Here's the drawing with two shaded views (mm, measured from the low corner). I have some questions. Coordinates: 2 decimals unless noted, no trailing zeros. Order: outer loops, then holes, each group sorted by start corner. A loop starts at its lowest first (then second) coordinate and runs counter-clockwise, first axis right, second up. Notation, with made-up numbers: (12, 28.5) - (56, 28.5) arc R5 cw to (56, 37.5) - close; hole circle Ø3 at (-33.5, 2). An arc over 180 degrees is marked (long way). Answer as a JSON object with one key per item and string values. Group by question number.
(1) Imagine slicing it at A-A, the plane x = 33.5. Write out the boundary of the cut face in (y, z).
(2) Will these pins go through, and if not, where does the flat tip stop? P1, Ø0.7, axis at x = 33.5, z = 7.6, coming from the -Y side; P2, Ø0.6, axis at x = 33.5, z = 30, coming from the -Y side.
(3) Imagine slicing it at B-B, the plane z = 30.4. Write out the boundary of the cut face in (x, y).
(4) Please list where these lines run through material, in increasing order: probe 1 along X at (y, z) = (0.65, 30.4); probe 2 along X at (y, z) = (1.8, 7.6); probe 3 along Z at (x, y) = (33.5, 1).
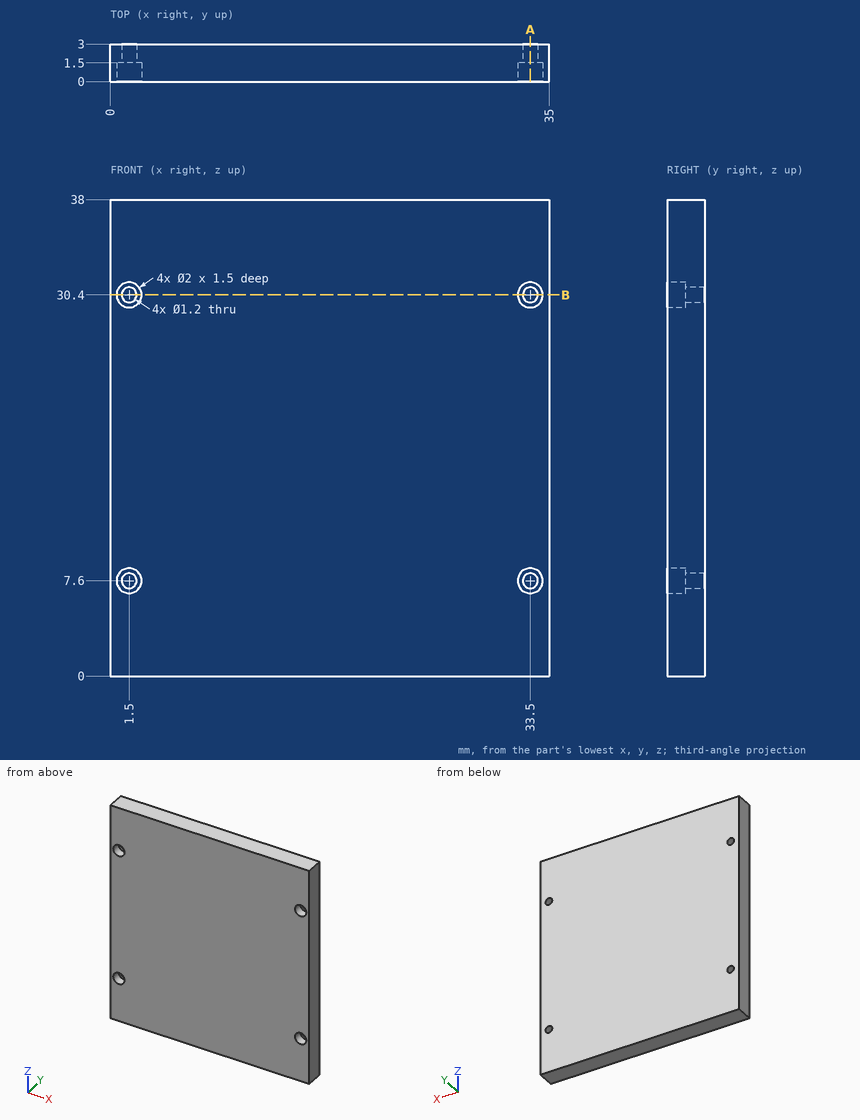
Result set:
{
 "1": {"outline": "(0, 0) - (3, 0) - (3, 7) - (1.5, 7) - (1.5, 6.6) - (0, 6.6) - close; (0, 8.6) - (1.5, 8.6) - (1.5, 8.2) - (3, 8.2) - (3, 29.8) - (1.5, 29.8) - (1.5, 29.4) - (0, 29.4) - close; (0, 31.4) - (1.5, 31.4) - (1.5, 31) - (3, 31) - (3, 38) - (0, 38) - close"},
 "2": {"P1": "passes through", "P2": "stops at y = 1.5"},
 "3": {"outline": "(0, 0) - (0.5, 0) - (0.5, 1.5) - (0.9, 1.5) - (0.9, 3) - (0, 3) - close; (2.1, 1.5) - (2.5, 1.5) - (2.5, 0) - (32.5, 0) - (32.5, 1.5) - (32.9, 1.5) - (32.9, 3) - (2.1, 3) - close; (34.1, 1.5) - (34.5, 1.5) - (34.5, 0) - (35, 0) - (35, 3) - (34.1, 3) - close"},
 "4": {"probe 1": "x = 0 to 0.5, 2.5 to 32.5, 34.5 to 35", "probe 2": "x = 0 to 0.9, 2.1 to 32.9, 34.1 to 35", "probe 3": "z = 0 to 6.6, 8.6 to 29.4, 31.4 to 38"}
}
